Part model, mm, in its own coordinate system. A direction names the side the tool comes from. Give positions to 0.01 mm unless a question says otherwise; leave off trailing zeros. Write each loop counter-clockwise with the first axis right and the second up, starting at its lowest first coordinate (ties: lowest second). Pieces come first, ordered by that corner, then holes. Notation, with made-up numbers: (41, 63.5) - (77, 63.5) arc R24 ccw to (77, 90.5) - close; hole circle Ø10 at (-25, 68). An arc over 180 degrees is marked (long way). Answer in a Markdown table with one row per item. Add a question column.
1. Probe line 1 along X through (y, z) = (-21, -9.5); line 2 along X through (y, z) = (-12, 12.5); line 3 along Z through (x, y) = (24.5, 9.5). List the from-to ranges inside material, lowest first.
2. Band-saw the part on B-B on z = 7. Write the cut outline in (x, y), plus the area to 3 significant figures.
3. Band-saw the part on A-A on y = -24. Write the cut outline in (x, z).
4. Band-saw the part on C-C on x = 24.5. Write the cut outline in (y, z), plus the area to 3 significant figures.
5. Which spindle directions (+Z, -Z, +X, -X, +Y, -Y) get a long thin tool onto all of the face, cutting with end or side? Do faces 1 (the flat face through (10, 0, 9)), 2 (the flat face through (23, -3, 0)), 3 (the flat face through (0, 10, 9)), 4 (the flat face through (38.1, 0, 9)). Say none if no direction does.
6. Drop flat-ended pins along their axis: pin 1 Ø15 at (y, z) = (3.5, 14) entering from +X; pin 2 Ø21 at (y, z) = (-15.5, 8) entering from -X; pin 3 Ø21 at (x, z) = (9.5, 5) entering from -Y; pin 4 Ø21 at (y, z) = (-25.5, -12) entering from -X. Give the stop position or say it passes through.
7. Band-saw the part on D-D on y = -7. Write the cut outline in (x, z).
```python
from build123d import *

# Parameters (mm, degrees)
F1_DEPTH = 19.05
F2_W     = 19.05
F2_H     = 19.05
F3_DEPTH = 19.05


with BuildPart() as f1:
    # F0 (on Top) → F1 (new body)
    with BuildSketch(Plane.XY):
        Polygon((0, 19.05), (0, 0), (19.400613, 0), (19.400613, -38.1), (57.500613, -38.1), (57.500613, -19.05), (38.1, -19.05), (38.1, 19.05), align=None)
    extrude(amount=F1_DEPTH)

    # F2 (on face) → F3 (join)
    with BuildSketch(Plane(origin=(0, 0, 0), x_dir=(1, 0, 0), z_dir=(0, 0, -1))):
        with Locations((47.975613, 28.575)):
            Rectangle(F2_W, F2_H)
    extrude(amount=F3_DEPTH)


solid = f1.part
```
Values:
| question | item | result |
|---|---|---|
| 1 | line 1 | x = 38.45 to 57.5 |
| 1 | line 2 | x = 19.4 to 38.1 |
| 1 | line 3 | z = 0 to 19.05 |
| 2 | outline | (0, 0) - (19.4, 0) - (19.4, -38.1) - (57.5, -38.1) - (57.5, -19.05) - (38.1, -19.05) - (38.1, 19.05) - (0, 19.05) - close |
| 2 | area | 1,810 mm² |
| 3 | outline | (19.4, 0) - (38.45, 0) - (38.45, -19.05) - (57.5, -19.05) - (57.5, 19.05) - (19.4, 19.05) - close |
| 4 | outline | (-38.1, 0) - (19.05, 0) - (19.05, 19.05) - (-38.1, 19.05) - close |
| 4 | area | 1,090 mm² |
| 5 | face 1 | +Z, -Z, -X, -Y |
| 5 | face 2 | -Z, -X, +Y, -Y |
| 5 | face 3 | +Z, -Z, -X, +Y, -Y |
| 5 | face 4 | +Z, -Z, +X, +Y |
| 6 | pin 1 | stops at x = 38.1 |
| 6 | pin 2 | stops at x = 19.4 |
| 6 | pin 3 | stops at y = -38.1 |
| 6 | pin 4 | stops at x = 38.45 |
| 7 | outline | (19.4, 0) - (38.1, 0) - (38.1, 19.05) - (19.4, 19.05) - close |
